Part model, mm, in its own coordinate system. A direction names the side the tool comes from. Give positions to 0.01 mm unless a question says otherwise; leave off trailing zeros. Loops run counter-clockwise (first coordinate to the right, second up) from the corner with the lowest first, then second, coordinate; pieces in that order, holes last. Notation, with made-up numbers: (-38.75, 34) -> (4.25, 34) arc R6 cw to (4.25, 38) -> close; hole circle Ø8 at (88, 30). An arc over 180 degrees is marked (long way). Write item = value, one per line.
Autodesk Fusion 360 part; units mm, degrees
sketch "Sketch1" plane through (0, 0, 0) normal (0, 0, 1) x (1, 0, 0)
  line L0 (1.5, 2) -> (-1.5, 2)
  arc A0 (-1.5, 2) -> (1.5, 2) centre (0, 0) ccw
cylinder "CylinderPrimitive1" add diameter 80 height 5 placed x (1, 0, 0) y (0, 1, 0) z (0, 0, 1) at (0, 0, 0) makes body 1
cylinder "CylinderPrimitive2" add diameter 20 height 30 placed x (1, 0, 0) y (0, 1, 0) z (0, 0, 1) at (0, 0, 5) bodies 1
extrude "Extrude1" cut sketch "Sketch1" along normal blind 44 bodies 1
fillet "Fillet1" radius 4 1 edges at (-37.2931, -14.4646, 5) on bodies 1
sketch "Sketch4" plane through (0, 0, 35) normal (0, 0, 1) x (-1, 0, 0)
  line L0 (1.5, -2) -> (-1.5, -2)
  arc A0 (1.5, -2) -> (-1.5, -2) centre (0, 0) ccw
  circle A1 centre (0, 0) radius 10
cylinder "CylinderPrimitive3" add diameter 4.5 height 31 placed x (1, 0, 0) y (0, 0, -1) z (0, 1, 0) at (0, 0, 10) separate body makes body 2
move_body "Move1" bodies 2 to x (1, 0, 0) y (0, 1, 0) z (0, 0, 1) at (0, -16, 0)
combine "Combine1" operation cut target body 1 tool bodies 2
1) Drop flat-ended pins along their axis: P1, Ø8, axis at x = -26, z = 5.5, coming from the +Y side; P2, Ø6, axis at y = 17, z = 4.5, coming from the -X side; P3, Ø3, axis at x = 23, z = 4.5, coming from the +Y side. Give the stop position or say it passes through.
Resolved:
P1 = 32.17
P2 = -36.87
P3 = 32.46
2) Slice it at A-A, the plane y = 0. List the corners of the cut face in (x, z), and give its area (3 significant figures).
Resolved:
outline = (-40, 0) -> (-2.5, 0) -> (-2.5, 35) -> (-10, 35) -> (-10, 5) -> (-36, 5) arc R4 ccw to (-40, 1) -> close; (2.5, 0) -> (40, 0) -> (40, 1) arc R4 ccw to (36, 5) -> (10, 5) -> (10, 35) -> (2.5, 35) -> close
area = 818 mm²
3) Pull direction X, two halves, no side cores. Call faces 1 (the face through (-0.1, 2.4, 35)), 2 (the face through (2.146, 5.607, 9.324)), 3 (the face through (9.54, 3, 20.21)): pulls with the +X half, pulls with the -X half, needs draft (parallel to the pull), parting line crosses it, or undercut.
Resolved:
face_1 = needs draft
face_2 = undercut
face_3 = parting line crosses it
4) Which spindle directions (+Z, -Z, +X, -X, +Y, -Y) get a long thin tool onto all of the face, cutting with end or side? Do faces 4 (the face through (7.5, -7.5, 5)), 5 (the face through (0, 2, 23)), 6 (the face through (2.146, -5.482, 9.324)). Say none if no direction does.
Resolved:
face_4 = +Z
face_5 = +Z, -Z
face_6 = +Y, -Y
5) Slice it at B-B, the plane x = 0. List the corners of the cut face in (y, z), and give its area (3 significant figures).
Resolved:
outline = (-40, 0) -> (-2.5, 0) -> (-2.5, 7.75) -> (-10, 7.75) -> (-10, 5) -> (-36, 5) arc R4 ccw to (-40, 1) -> close; (-10, 12.25) -> (-2.5, 12.25) -> (-2.5, 35) -> (-10, 35) -> close; (2, 0) -> (40, 0) -> (40, 1) arc R4 ccw to (36, 5) -> (10, 5) -> (10, 7.75) -> (2, 7.75) -> close; (2, 12.25) -> (10, 12.25) -> (10, 35) -> (2, 35) -> close
area = 766 mm²
6) Drill centre lines: line 1 along Z through (x, y) = (0, -6.75); line 2 along Z through (x, y) = (-9.5, -19); line 3 along Y through (x, z) = (0, 23). Where is each one in solid material? Low to high. Write a range as [from, to].
Resolved:
line_1 = [0, 7.75], [12.25, 35]
line_2 = [0, 5]
line_3 = [-10, -2.5], [2, 10]
7) Slice it at C-C, the plane z = 10. List the corners of the cut face in (x, y), and give its area (3 significant figures).
Resolved:
outline = (-2.25, -9.74) -> (-2.25, -1.09) arc R2.5 cw to (-2.25, 1.09) -> (-2.25, 9.74) arc R10 ccw to start; (2.25, -9.74) arc R10 ccw to (2.25, 9.74) -> (2.25, 1.09) arc R2.5 cw to (2.25, -1.09) -> close
area = 224 mm²
8) Slice it at D-D, the plane z = 3.5. List the corners of the cut face in (x, y) (1 decimal), and give its area (3 significant figures).
Resolved:
outline = circle Ø78.2 at (0, 0); hole (-1.5, 2) arc R2.5 ccw (long way) to (1.5, 2) -> close
area = 4,790 mm²
